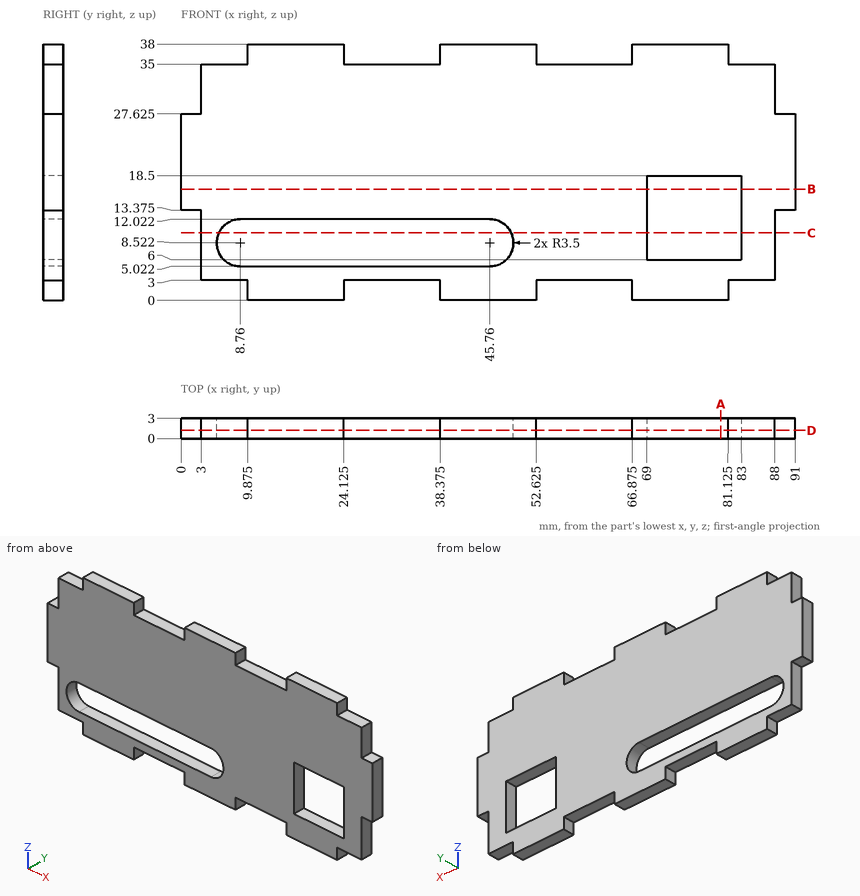
Job drawing, mm, ordinate dimensions from the low corner. One solid piece. Give positions to 0.01 mm unless a question says otherwise; leave off trailing zeros. Loops run counter-clockwise (first coordinate to the right, second up) from the corner with the lowest first, then second, coordinate; pieces in that order, holes last. Notation, with made-up numbers: M 87,20.25 L 117,20.25 A24 ccw 117,45.25 Z; hole C 28,62.25 d7. An arc over 180 degrees is marked long. Put each result on its own line as item: value. Start each with the question number.
1) Saw through at D-D (y = 1.2). State how many separate pieces and enclosed holes the cut face has, then the cut area to 3 significant figures.
2) Saw through at C-C (z = 10). List the corners of the cut face in (x, y).
3) Saw through at A-A (x = 80). List the corners of the cut face in (y, z), then the cut area to 3 significant figures.
4) Saw through at B-B (z = 16.5). List the corners of the cut face in (x, y).
5) Probe probe 1 along X at (y, z) = (1.55, 36.5) (3 decimals); probe 2 along X at (y, z) = (2.1, 8.5); probe 3 along Z at (x, y) = (29, 2.85). List the from-to ranges inside material, lowest first.
6) Flat gauge pins, fed straight in: pin 1 (0.9 mm diameter, centred on y = 1, z = 37, fed in from +X) (3 decimals); pin 2 (1 mm diameter, centred on x = 61, y = 0.5, fed in from -Z); pin 3 (0.9 mm diameter, centred on y = 1, z = 1, fed in from -X) (3 decimals). Where does each tip first touch, or does it go through?
Numbers:
1. separate pieces: 1
1. enclosed holes: 2
1. area: 2,590 mm^2
2. outline: M 3,0 L 5.59,0 L 5.59,3 L 3,3 Z; M 48.93,0 L 69,0 L 69,3 L 48.93,3 Z; M 83,0 L 88,0 L 88,3 L 83,3 Z
3. outline: M 0,0 L 3,0 L 3,6 L 0,6 Z; M 0,18.5 L 3,18.5 L 3,38 L 0,38 Z
3. area: 76.5 mm^2
4. outline: M 0,0 L 69,0 L 69,3 L 0,3 Z; M 83,0 L 91,0 L 91,3 L 83,3 Z
5. probe 1: 9.875 to 24.125, 38.375 to 52.625, 66.875 to 81.125
5. probe 2: 3 to 5.26, 49.26 to 69, 83 to 88
5. probe 3: 3 to 5.02, 12.02 to 35
6. pin 1: x = 81.125
6. pin 2: z = 3
6. pin 3: x = 9.875
